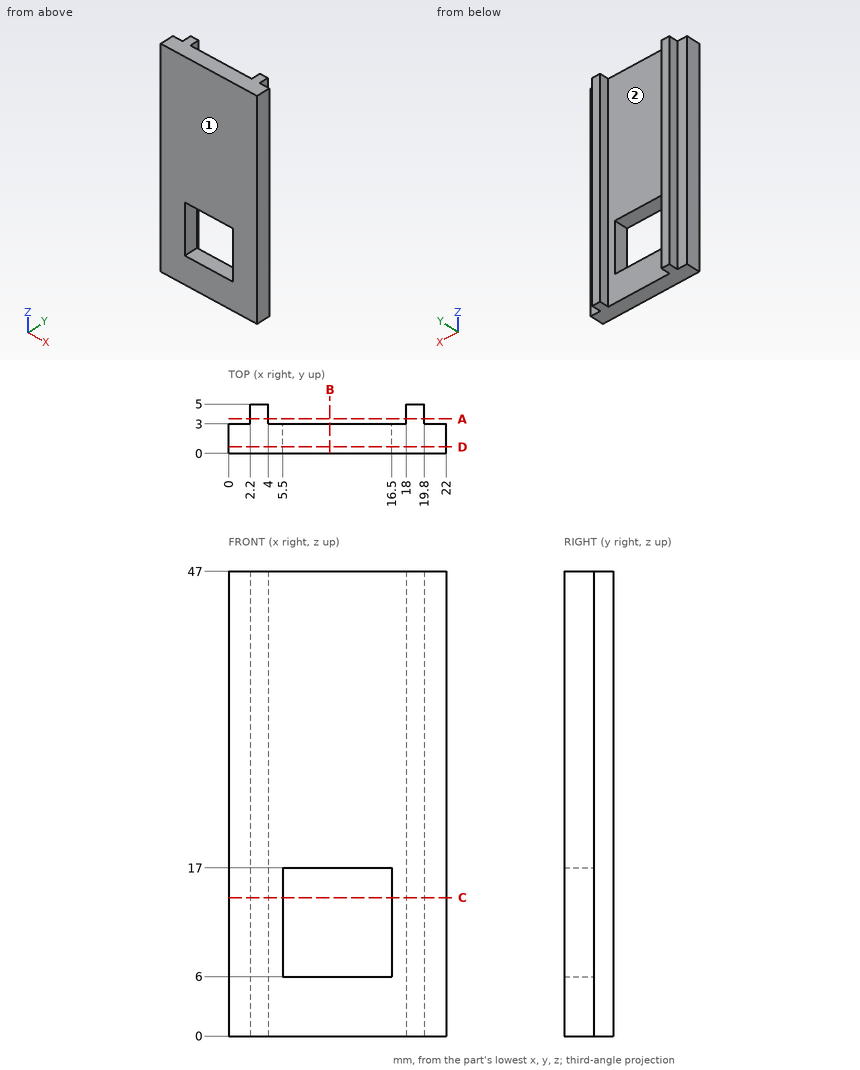
Part print with two shaded views. Sizes in mm from the minimum x, y, z corner. Round coordinates to 2 decimals unless told otherwise and drop trailing zeros. Loops run counter-clockwise (first coordinate to the right, second up) from the corner with the lowest first, then second, coordinate; pieces in that order, holes last.
Item 1: Saw through at D-D (y = 0.65). List the corners of the cut face in (x, z), then the cut area to 3 significant figures.
Item 2: Saw through at A-A (y = 3.5). List the corners of the cut face in (x, z).
Item 3: Drill centre lines: line 1 along X through (y, z) = (3.75, 36); line 2 along Z through (x, y) = (9.75, 0.75); line 3 along X through (y, z) = (1.85, 13). Where is each one in solid material? Low to high.
Item 4: Saw through at C-C (z = 14). List the corners of the cut face in (x, y).
Item 5: Saw through at B-B (x = 10.25). List the corners of the cut face in (y, z), then the cut area to 3 significant figures.
Item 6: Two-plate mould, pull along X, no slides. Class the marked faces 1 and 2: released by +X, released by -X, zero draft, split by the parting line, or undercut.
Item 7: Pin check, flat tips, straight feed: P1, Ø0.6, axis at y = 4.5, z = 29, coming from the -X side; P2, Ø2, axis at y = 4.5, z = 14, coming from the +X side; P3, Ø0.7, axis at x = 21, z = 35, coming from the +Y side. Stop position of each tip, or through.
Worked answers:
1. outline: (0, 0) - (22, 0) - (22, 47) - (0, 47) - close; hole (5.5, 6) - (16.5, 6) - (16.5, 17) - (5.5, 17) - close
1. area: 913 mm2
2. outline: (2.2, 0) - (4, 0) - (4, 47) - (2.2, 47) - close; (18, 0) - (19.8, 0) - (19.8, 47) - (18, 47) - close
3. line 1: x = 2.2 to 4, 18 to 19.8
3. line 2: z = 0 to 6, 17 to 47
3. line 3: x = 0 to 5.5, 16.5 to 22
4. outline: (0, 0) - (5.5, 0) - (5.5, 3) - (4, 3) - (4, 5) - (2.2, 5) - (2.2, 3) - (0, 3) - close; (16.5, 0) - (22, 0) - (22, 3) - (19.8, 3) - (19.8, 5) - (18, 5) - (18, 3) - (16.5, 3) - close
5. outline: (0, 0) - (3, 0) - (3, 6) - (0, 6) - close; (0, 17) - (3, 17) - (3, 47) - (0, 47) - close
5. area: 108 mm2
6. face 1: zero draft
6. face 2: undercut
7. P1: stops at x = 2.2
7. P2: stops at x = 19.8
7. P3: stops at y = 3
